Could you check a few things on this model? Use its own coordinates, in mm. A direction names the side the tool comes from. Coordinates: 2 decimals unless noted, no trailing zeros. One line per item, written item: value. Start each with the question number.
(1) On a 3-axis mill with a long thin cutter (end or side, diameter ignored), from which of +Z, -Z, +X, -X, +Y, -Y can I reach the whole of each face in a straight line? I mean faces 3 (the face through (1.08, 4.88, 4.67)), 4 (the face through (-1, -21, 8)). Say none if no direction works.
(2) If I drill on line 1 along Z through (x, y) = (29.5, 85); line 2 along Y through (x, z) = (0, 5); line 3 along Y through (x, z) = (-79.5, 17.5), over which ranges is the centre line in solid material (lowest first)? Write a range as from..to.
(3) If we mould it in two halves opening along X, with no side actions, what happens to faces 1 (the face through (95.38, 30.04, 17.84)), 2 (the face through (20, 1, 0))? For each: pulls with the +X half, pulls with the -X half, needs draft (parallel to the pull), parting line crosses it, or undercut.
(4) I'm going to push flat-ended pins straight in: P1, Ø3, axis at y = 36, z = 5, coming from the -X side; P2, Ø2, axis at y = 65, z = 5.5, coming from the +X side; P3, Ø2, axis at x = -41, z = 23.5, coming from the +Y side. Where does each tip first touch, or does it pass through?
```python
from build123d import *

# Parameters (mm, degrees)
F0_R           = 110
F1_DEPTH       = 28
F2_R           = 13.99999
F3_R           = 100
F4_DEPTH       = 20
F6_D           = 10
F6_CSINK_D     = 12.5
F6_CSINK_ANGLE = 90


# Not quite as in the source:
# - a fillet or chamfer is up to 0.001 mm smaller than in the source, because OpenCascade refuses the exact size


with BuildPart() as f1:
    # F0 (on Top) → F1 (new body)
    with BuildSketch(Plane.XY):
        Circle(F0_R)
    extrude(amount=F1_DEPTH)

    # F2 (radius 14 in the source; OpenCascade refuses exactly that, so slightly less here)
    f2_edges = [f1.edges().sort_by_distance(p)[0] for p in [
        (-110, 0, 28),
        (-110, 0, 0),
    ]]
    fillet(f2_edges, radius=F2_R)

    # F3 (on face) → F4 (cut)
    with BuildSketch(Plane.XY.offset(28)):
        Circle(F3_R)
    extrude(amount=-F4_DEPTH, mode=Mode.SUBTRACT)

    # F6 (through all)
    with Locations(Plane(origin=(0, 0, 0), x_dir=(1, 0, 0), z_dir=(0, 0, -1))):
        with Locations((0, 0)):
            CounterSinkHole(F6_D / 2, F6_CSINK_D / 2, counter_sink_angle=F6_CSINK_ANGLE)


solid = f1.part
```
Values:
1. face 3: +Z, -Z
1. face 4: +Z
2. line 1: z = 0..8
2. line 2: y = -106.72..-5, 5..106.72
2. line 3: y = -75.38..-60.66, 60.66..75.38
3. face 1: undercut
3. face 2: needs draft
4. P1: stops at x = -101.76
4. P2: stops at x = 86.32
4. P3: stops at y = 99.06
